Can you work these out from the model? Positions are in its coordinate system, mm. Face numbers are marked on the shaded views. A direction names the side the tool comes from. Coordinates: 2 decimals unless noted, no trailing zeros. Order: outer loops, then holes, each group sorted by start corner. A loop starts at its lowest first (then second) coordinate and runs counter-clockwise, first axis right, second up. Notation, with made-up numbers: (77, -8.5) -> (132, -8.5) arc R24 ccw to (132, 27.5) -> close; hole circle Ø5 at (57, 77). An arc over 180 degrees is marked (long way). Use a Markdown table: item, result. Add a question column.
1. For the marked faces 1 and 2, which set-ups out of +Z, -Z, +X, -X, +Y, -Y let a thin tool reach every point of the face, with its end or its side?
2. We'd pull the mould along Y, two halves only. Please class the marked faces 3, 4 and 5: pulls with the +Y half, pulls with the -Y half, needs draft (parallel to the pull), parting line crosses it, or undercut.
3. If I drill on line 1 along X through (y, z) = (1, 51.5); line 2 along Y through (x, z) = (-20.5, 60.5); line 3 along Z through (x, y) = (36, 1.5), over which ranges is the centre line in solid material (lowest first)? Write a range as from..to.
4. Suppose I cut it at D-D, the plane z = 7. List the corners of the cut face in (x, y) for me, then the cut area to 3 significant figures.
5. For pin 1 Ø1.5 at (x, z) = (10, 48.5) entering from -Y; pin 2 Ø14 at (x, z) = (15.5, 56) entering from -Y; pin 3 Ø10 at (x, y) = (-16, -11) entering from +Z, each with a flat end and sliding along its axis, tell me the tip position at first contact or that it passes through.
6. Suppose I cut it at B-B, the plane x = 28.5. List the corners of the cut face in (y, z) for me, then the cut area to 3 significant figures.
7. Suppose I cut it at C-C, the plane y = -20. List the corners of the cut face in (x, z) for me.
8. Suppose I cut it at A-A, the plane z = 33. List the corners of the cut face in (x, y) for me, then the cut area to 3 significant figures.
```python
from build123d import *

# Parameters (mm, degrees)
F0_W        = 76.2
F0_H        = 50.8
F1_DEPTH    = 50.8
F2_W        = 58.6486
F2_H        = 9.7282
F3_DEPTH    = 19.05
F5_DEPTH    = 76.2
F1_FACE_W   = 76.2
F1_FACE_H   = 25.4
F1_FACE_W_2 = 58.6486
F1_FACE_H_2 = 9.7282
F6_DEPTH    = 12.7


with BuildPart() as f1:
    # F0 (on Top) → F1 (new body)
    with BuildSketch(Plane.XY):
        with Locations((7.004574, -5.004832)):
            Rectangle(F0_W, F0_H)
    extrude(amount=F1_DEPTH)

    # F2 (on face) → F3 (cut)
    with BuildSketch(Plane.XY.offset(50.8)):
        with Locations((7.004574, 5.802868)):
            Rectangle(F2_W, F2_H)
    extrude(amount=-F3_DEPTH, mode=Mode.SUBTRACT)

    # F4 (on face) → F5 (cut)
    with BuildSketch(Plane(origin=(-31.095426, 0, 0), x_dir=(0, -1, 0), z_dir=(-1, 0, 0))):
        Polygon((30.404832, 50.8), (5.004832, 50.8), (30.404832, 0), align=None)
    extrude(amount=-F5_DEPTH, mode=Mode.SUBTRACT)

    # F1_face (on face) → F6 (join)
    with BuildSketch(Plane(origin=(7.004574, -5.004832, 50.8), x_dir=(1, 0, 0), z_dir=(0, 0, 1))):
        with Locations((0, 12.7)):
            Rectangle(F1_FACE_W, F1_FACE_H)
        with Locations((0, 10.8077)):
            Rectangle(F1_FACE_W_2, F1_FACE_H_2, mode=Mode.SUBTRACT)
    extrude(amount=F6_DEPTH)


solid = f1.part
```
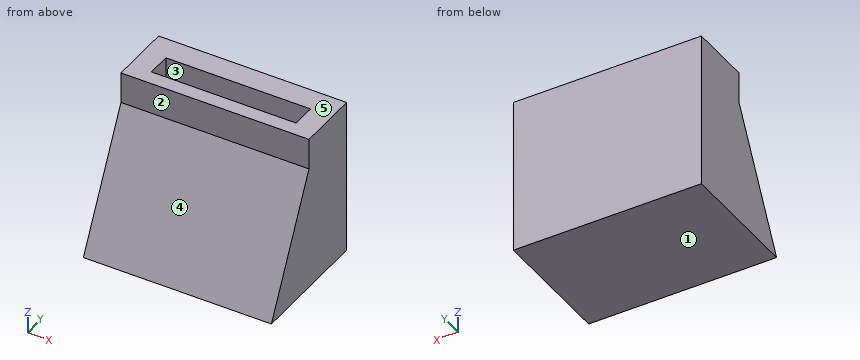
Worked out:
| question | item | result |
|---|---|---|
| 1 | face 1 | -Z, +X, -X, +Y, -Y |
| 1 | face 2 | +Z, +X, -X, -Y |
| 2 | face 3 | undercut |
| 2 | face 4 | pulls with the -Y half |
| 2 | face 5 | needs draft |
| 3 | line 1 | x = -31.1..-22.32, 36.33..45.1 |
| 3 | line 2 | y = -5..0.94, 10.67..20.4 |
| 3 | line 3 | z = 0..31.75 |
| 4 | outline | (-31.1, -26.9) -> (45.1, -26.9) -> (45.1, 20.4) -> (-31.1, 20.4) -> close |
| 4 | area | 3,600 mm² |
| 5 | pin 1 | stops at y = -6.53 |
| 5 | pin 2 | stops at y = -5.9 |
| 5 | pin 3 | stops at z = 48.81 |
| 6 | outline | (-30.4, 0) -> (20.4, 0) -> (20.4, 63.5) -> (10.67, 63.5) -> (10.67, 31.75) -> (0.94, 31.75) -> (0.94, 63.5) -> (-5, 63.5) -> (-5, 50.8) -> close |
| 6 | area | 1,950 mm² |
| 7 | outline | (-31.1, 0) -> (45.1, 0) -> (45.1, 20.81) -> (-31.1, 20.81) -> close |
| 8 | outline | (-31.1, -13.9) -> (45.1, -13.9) -> (45.1, 20.4) -> (-31.1, 20.4) -> close; hole (-22.32, 0.94) -> (36.33, 0.94) -> (36.33, 10.67) -> (-22.32, 10.67) -> close |
| 8 | area | 2,040 mm² |
